```python
from build123d import *

# Parameters (mm, degrees)
MODEL_R                 = 27
MODEL_R_2               = 1.5
SALIENTE_EXTRUIR1_DEPTH = 3


with BuildPart() as part:
    # Model → Saliente-Extruir1 (new body)
    with BuildSketch(Plane.XY):
        with Locations((158.427277744, 241.952019993)):
            Circle(MODEL_R)
        with Locations((158.427277744, 262.076631791)):
            Circle(MODEL_R_2, mode=Mode.SUBTRACT)
        with Locations((140.998852686, 252.014325892)):
            Circle(MODEL_R_2, mode=Mode.SUBTRACT)
        with Locations((140.998852686, 231.889714094)):
            Circle(MODEL_R_2, mode=Mode.SUBTRACT)
        with Locations((158.427277744, 221.827408196)):
            Circle(MODEL_R_2, mode=Mode.SUBTRACT)
        with Locations((175.855702802, 231.889714094)):
            Circle(MODEL_R_2, mode=Mode.SUBTRACT)
        with Locations((175.855702802, 252.014325892)):
            Circle(MODEL_R_2, mode=Mode.SUBTRACT)
        Polygon((174.352685576, 246.268428845), (180.425586348, 241.679222344), (170.128101379, 230.318416671), (169.190182352, 222.764527077), (154.202693546, 226.002007819), (147.191873748, 223.037324726), (142.501869912, 237.635611142), (136.427281639, 242.226092863), (146.726454109, 253.585623316), (147.664373136, 261.139512909), (162.651861941, 257.902032168), (169.66268174, 260.86671526), align=None, mode=Mode.SUBTRACT)
    extrude(amount=SALIENTE_EXTRUIR1_DEPTH)


solid = part.part
```
Work out the finished part from the listing and answer in its coordinate system (mm). Round coordinates to 2 decimals unless told otherwise and drop trailing zeros. Write each loop counter-clockwise with the first axis right and the second up, starting at its lowest first coordinate (ties: lowest second). Pieces come first, ordered by that corner, then holes.
1) A cutting plane is placed at D-D on x = 165.5. Determine the outline of the cut face in (y, z), and give its area (3 significant figures).
2) Determine the mould class of faces 1 (the face through (131.453, 243.139, 1.479)), 2 (the face through (144.88, 230.23, 1.48)), 3 (the face through (158, 224, 0)) for opening direction Y: pulls with the +Y half, pulls with the -Y half, needs draft (parallel to the pull), parting line crosses it, or undercut.
3) A cutting plane is placed at A-A on y = 248. Determine the outline of the cut face in (x, z).
4) A flat-ended cylindrical pin translates along its axis: P1, Ø3.5, axis at x = 158.43, y = 262.08, coming from the -Z side. Find the tip coordinate at first contact, or state that the pin passes through.
5) A cutting plane is placed at C-C on z = 2.15. Determine the outline of the cut face in (x, y).
6) A cutting plane is placed at B-B on x = 176. Determine the outline of the cut face in (y, z), and give its area (3 significant figures).
7) Consider probe 1 along Y at (x, z) = (142, 1.9); probe 2 along Y at (x, z) = (177, 2); probe 3 along X at (y, z) = (255, 1.2). Determine where each line is inside the solid, lowest interval first.
Entries:
1. outline: (215.89, 0) - (223.56, 0) - (223.56, 3) - (215.89, 3) - close; (259.11, 0) - (268.01, 0) - (268.01, 3) - (259.11, 3) - close
1. area: 49.7 mm2
2. face 1: parting line crosses it
2. face 2: undercut
2. face 3: needs draft
3. outline: (132.11, 0) - (141.66, 0) - (141.66, 3) - (132.11, 3) - close; (173.8, 0) - (184.74, 0) - (184.74, 3) - (173.8, 3) - close
4. P1: stops at z = 0
5. outline: circle Ø54 at (158.43, 241.95); hole (136.43, 242.23) - (142.5, 237.64) - (147.19, 223.04) - (154.2, 226) - (169.19, 222.76) - (170.13, 230.32) - (180.43, 241.68) - (174.35, 246.27) - (169.66, 260.87) - (162.65, 257.9) - (147.66, 261.14) - (146.73, 253.59) - close; hole circle Ø3 at (141, 231.89); hole circle Ø3 at (141, 252.01); hole circle Ø3 at (158.43, 221.83); hole circle Ø3 at (158.43, 262.08); hole circle Ø3 at (175.86, 231.89); hole circle Ø3 at (175.86, 252.01)
6. outline: (221.45, 0) - (230.4, 0) - (230.4, 3) - (221.45, 3) - close; (233.38, 0) - (236.8, 0) - (236.8, 3) - (233.38, 3) - close; (245.02, 0) - (250.52, 0) - (250.52, 3) - (245.02, 3) - close; (253.51, 0) - (262.45, 0) - (262.45, 3) - (253.51, 3) - close
6. area: 80.4 mm2
7. probe 1: y = 220.52 to 230.77, 233.01 to 238.01, 248.37 to 250.9, 253.13 to 263.38
7. probe 2: y = 222.35 to 230.92, 232.86 to 237.9, 244.27 to 251.04, 252.98 to 261.55
7. probe 3: x = 134.79 to 146.9, 171.55 to 182.07
